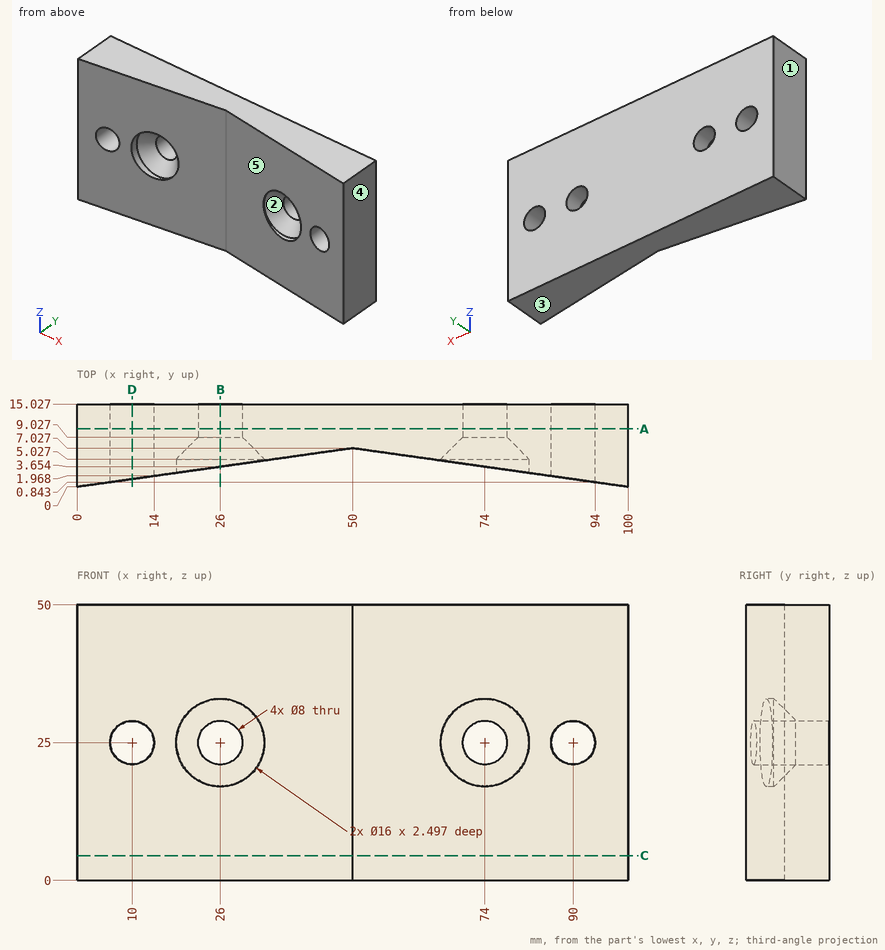
Print and shaded views of the part. All mm, measured from the part's lowest x, y and z. A direction names the side the tool comes from. Round coordinates to 2 decimals unless told otherwise and drop trailing zeros. Write each loop counter-clockwise with the first axis right and the second up, starting at its lowest first coordinate (ties: lowest second). Pieces come first, ordered by that corner, then holes. Notation, with made-up numbers: (60.5, 67.25) -> (88.5, 67.25) arc R10 cw to (88.5, 71.25) -> close; hole circle Ø5 at (-23.5, -40). An arc over 180 degrees is marked (long way). Write item = value, one per line.
(1) Tool access for the marked faces 4 and 5: list every direction of +Z, -Z, +X, -X, +Y, -Y with a clear straight run to the whole face (end or side of a thin tool).
Answer:
face_4 = +Z, -Z, +X, +Y, -Y
face_5 = +Z, -Z, -Y
(2) Band-saw the part on C-C (z = 4.5). Give the cut face in (x, y).
Answer:
outline = (0, 0) -> (50, 7.03) -> (100, 0) -> (100, 15.03) -> (0, 15.03) -> close
(3) Probe L1, parallel to X at y = 4.4, z = 25; L2, parallel to X at y = 11.1, z = 25; L3, parallel to Z at x = 26, y = 10.75. List the from-to ranges inside material, lowest first.
Answer:
L1 = 0 to 6, 14 to 18, 82 to 86, 94 to 100
L2 = 0 to 6, 14 to 22, 30 to 70, 78 to 86, 94 to 100
L3 = 0 to 21, 29 to 50
(4) Band-saw the part on A-A (y = 10.5). Give the cut face in (x, z).
Answer:
outline = (0, 0) -> (100, 0) -> (100, 50) -> (0, 50) -> close; hole circle Ø8 at (10, 25); hole circle Ø8 at (26, 25); hole circle Ø8 at (74, 25); hole circle Ø8 at (90, 25)
(5) Band-saw the part on D-D (x = 10). Give the cut face in (y, z) (1 decimal), then the cut area to 3 significant figures.
Answer:
outline = (1.4, 0) -> (15, 0) -> (15, 21) -> (1.4, 21) -> close; (1.4, 29) -> (15, 29) -> (15, 50) -> (1.4, 50) -> close
area = 572 mm2
(6) Band-saw the part on B-B (x = 26). Give the cut face in (y, z).
Answer:
outline = (3.65, 0) -> (15.03, 0) -> (15.03, 21) -> (9.03, 21) -> (5.03, 17) -> (3.65, 17) -> close; (3.65, 33) -> (5.03, 33) -> (9.03, 29) -> (15.03, 29) -> (15.03, 50) -> (3.65, 50) -> close
(7) Two-plate mould, pull along Z, no slides. Class the marked faces 1, 2 and 3: pulls with the +Z half, pulls with the -Z half, needs draft (parallel to the pull), parting line crosses it, or undercut.
Answer:
face_1 = needs draft
face_2 = undercut
face_3 = pulls with the -Z half
(8) Flat gauge pins, fed straight in: pin 1 (5 mm diameter, centred on x = 74, z = 25, fed in from -Y); pin 2 (13 mm diameter, centred on x = 74, z = 25, fed in from +Y); pin 3 (12 mm diameter, centred on x = 73.5, z = 41.5, fed in from -Y); pin 4 (4 mm diameter, centred on x = 41, z = 42.5, fed in from -Y). Where does each tip first touch, or does it go through?
Answer:
pin_1 = through
pin_2 = 15.03
pin_3 = 2.88
pin_4 = 5.48
